Geometry check sheet. Reference: drawing and pictorial views, mm from the part's lowest x, y, z. A direction names the side the tool comes from. Give positions to 0.01 mm unless a question says otherwise; leave off trailing zeros. Order: outer loops, then holes, each group sorted by start corner. A loop starts at its lowest first (then second) coordinate and runs counter-clockwise, first axis right, second up. Notation, with made-up numbers: (35, 32.5) - (77, 32.5) arc R18 cw to (77, 49.5) - close; hole circle Ø4 at (75, 86.5). An arc over 180 degrees is marked (long way). Answer in a Markdown table with one row per item.
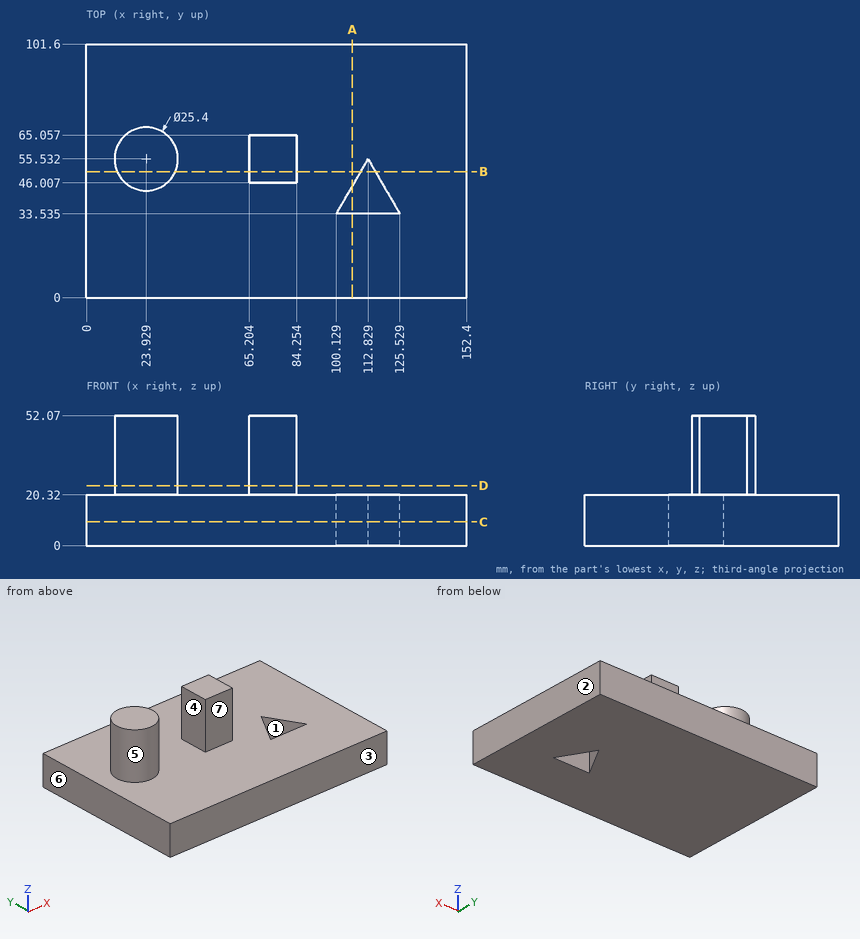
(1) Mould release check, pull along X, two halves, no side actions. Record for the marked faces 1, 2 and 3: pulls with the +X half, pulls with the -X half, needs draft (parallel to the pull), parting line crosses it, or undercut.
Geometry says:
| item | result |
|---|---|
| face 1 | undercut |
| face 2 | pulls with the +X half |
| face 3 | needs draft |
(2) Access from +Z, -Z, +X, -X, +Y, -Y to the whole of each face (thin tool, end or side, straight path). Record for the marked faces 4, 5, 6 and 7.
Geometry says:
| item | result |
|---|---|
| face 4 | +Z, +Y, -Y |
| face 5 | +Z |
| face 6 | +Z, -Z, -X, +Y, -Y |
| face 7 | +Z, +X, -Y |
(3) Thickness scan on L1, parallel to Z at x = 51, y = 67; L2, parallel to Y at x = 105, z = 8.5 (1 decimal); L3, parallel to Y at x = 112, z = 5.5 (1 decimal). Record the ranges inside material, lowest first.
Geometry says:
| item | result |
|---|---|
| L1 | 0 to 20.32 |
| L2 | 0 to 33.5, 42 to 101.6 |
| L3 | 0 to 33.5, 54.1 to 101.6 |
(4) Cross-section at D-D, the plane z = 24. Record the cut outline in (x, y) (1 decimal).
Geometry says:
| item | result |
|---|---|
| outline | circle Ø25.4 at (23.9, 55.5); (65.2, 46) - (84.3, 46) - (84.3, 65.1) - (65.2, 65.1) - close |
(5) Gauge pin test, flat ends, axial feed: P1, Ø8, axis at x = 74, z = 42.5, coming from the +Y side; P2, Ø1.5, axis at x = 32, z = 22.5, coming from the +Y side; P3, Ø5, axis at x = 17.5, z = 26.5, coming from the +Y side. Record the tip position at first contact, or that the pin passes through.
Geometry says:
| item | result |
|---|---|
| P1 | y = 65.06 |
| P2 | y = 65.91 |
| P3 | y = 67.61 |
(6) Cross-section at B-B, the plane y = 50.5. Record the cut outline in (x, z) (1 decimal), then the cut area to 3 significant figures.
Geometry says:
| item | result |
|---|---|
| outline | (0, 0) - (109.9, 0) - (109.9, 20.3) - (84.3, 20.3) - (84.3, 52.1) - (65.2, 52.1) - (65.2, 20.3) - (35.6, 20.3) - (35.6, 52.1) - (12.3, 52.1) - (12.3, 20.3) - (0, 20.3) - close; (115.7, 0) - (152.4, 0) - (152.4, 20.3) - (115.7, 20.3) - close |
| area | 4,320 mm² |
(7) Cross-section at C-C, the plane z = 9.5. Record the cut outline in (x, y) (1 decimal), then the cut area to 3 significant figures.
Geometry says:
| item | result |
|---|---|
| outline | (0, 0) - (152.4, 0) - (152.4, 101.6) - (0, 101.6) - close; hole (100.1, 33.5) - (125.5, 33.5) - (112.8, 55.5) - close |
| area | 15,200 mm² |
(8) Cross-section at A-A, the plane x = 106.5. Record the cut outline in (y, z) (1 decimal).
Geometry says:
| item | result |
|---|---|
| outline | (0, 0) - (33.5, 0) - (33.5, 20.3) - (0, 20.3) - close; (44.6, 0) - (101.6, 0) - (101.6, 20.3) - (44.6, 20.3) - close |
